```python
from build123d import *

# Parameters (mm, degrees)
CROQUIS1_R              = 450
CROQUIS1_R_2            = 448
SALIENTE_EXTRUIR2_DEPTH = 110
CROQUIS2_W              = 120
CROQUIS2_H              = 210
CROQUIS2_W_2            = 32
CROQUIS2_H_2            = 16.5
CORTAR_EXTRUIR2_DEPTH   = 500
CROQUIS3_W              = 120
CROQUIS3_H              = 66
CROQUIS3_W_2            = 32
CROQUIS3_H_2            = 16.5
CORTAR_EXTRUIR3_DEPTH   = 500


with BuildPart() as part:
    # Croquis1 → Saliente-Extruir2 (new body)
    with BuildSketch(Plane(origin=(0, 0, 0), x_dir=(1, 0, 0), z_dir=(0, 1, 0))):
        Circle(CROQUIS1_R)
        Circle(CROQUIS1_R_2, mode=Mode.SUBTRACT)
    extrude(amount=SALIENTE_EXTRUIR2_DEPTH)

    # Croquis2 → Cortar-Extruir2 (cut)
    with BuildSketch(Plane.XY):
        Rectangle(CROQUIS2_W, CROQUIS2_H)
        with Locations((-76, 8.25)):
            Rectangle(CROQUIS2_W_2, CROQUIS2_H_2)
        with Locations((76, 8.25)):
            Rectangle(CROQUIS2_W_2, CROQUIS2_H_2)
    extrude(amount=CORTAR_EXTRUIR2_DEPTH, mode=Mode.SUBTRACT)

    # Croquis3 → Cortar-Extruir3 (cut)
    with BuildSketch(Plane.XY):
        with Locations((0, 33)):
            Rectangle(CROQUIS3_W, CROQUIS3_H)
        with Locations((76, 8.25)):
            Rectangle(CROQUIS3_W_2, CROQUIS3_H_2)
        with Locations((-76, 8.25)):
            Rectangle(CROQUIS3_W_2, CROQUIS3_H_2)
    extrude(amount=-CORTAR_EXTRUIR3_DEPTH, mode=Mode.SUBTRACT)


solid = part.part
```
The model under review builds one solid part; all positions refer to its coordinate system, in mm. Round coordinates to 2 decimals unless told otherwise and drop trailing zeros. Order: outer loops, then holes, each group sorted by start corner. A loop starts at its lowest first (then second) coordinate and runs counter-clockwise, first axis right, second up. Notation, with made-up numbers: M 16.5,11.25 L 44.5,11.25 A9 ccw 44.5,28.25 Z; hole C 67.25,18 d7. An arc over 180 degrees is marked long. Use a Markdown table: item, result.
1) Insertion check: pin 1 (12 mm diameter, centred on y = 12, z = -106.5, fed in from -X); pin 2 (6 mm diameter, centred on y = 84, z = -201, fed in from +X); pin 3 (2.5 mm diameter, centred on x = 80, z = -442.5, fed in from -Y). Each pin has a flat end and moves straight along its axis. Give the tip position at first contact, or say it passes through.
Report:
| item | result |
|---|---|
| pin 1 | x = -438.63 |
| pin 2 | x = 404.1 |
| pin 3 | y = 16.5 |
2) Consider section B-B (x = 0). Write out the cut boundary in (y, z).
Report:
| item | result |
|---|---|
| outline | M 66,-450 L 110,-450 L 110,-448 L 66,-448 Z; M 105,448 L 110,448 L 110,450 L 105,450 Z |
3) Wall thickness on line 1 along X through (y, z) = (84.5, 0); line 2 along X through (y, z) = (30, -4); line 3 along Z through (x, y) = (75.5, 19): over which ranges is each line inside the solid? List them lowest first. Write a range as [from, to].
Report:
| item | result |
|---|---|
| line 1 | [-450, -448], [448, 450] |
| line 2 | [-449.98, -447.98], [447.98, 449.98] |
| line 3 | [-443.62, -441.59], [441.59, 443.62] |
4) Consider section A-A (y = 30). Write out the cut boundary in (x, z), then the cut area to 3 significant figures.
Report:
| item | result |
|---|---|
| outline | M -60,-445.98 L -60,-443.96 A448 cw -60,443.96 L -60,445.98 A450 ccw Z; M 60,-445.98 A450 ccw 60,445.98 L 60,443.96 A448 cw 60,-443.96 Z |
| area | 5,160 mm^2 |
5) Consider section C-C (y = 94.5). Write out the cut boundary in (x, z), then the cut area to 3 significant figures.
Report:
| item | result |
|---|---|
| outline | M -60,443.96 L -60,445.98 A450 ccw long 60,445.98 L 60,443.96 A448 cw long Z |
| area | 5,400 mm^2 |
6) Draft analysis for pull direction Z (two halves, no side actions). For faces 1 (the face through (-97.118, 54.23, 437.347)), 2 (the face through (-97.55, 54.23, 439.3)), state which applies: released by +Z, released by -Z, zero draft, split by the parting line, or undercut.
Report:
| item | result |
|---|---|
| face 1 | undercut |
| face 2 | split by the parting line |
